```python
from build123d import *

# Parameters (mm, degrees)
F1_DEPTH = 2
F2_DEPTH = 4


with BuildPart() as f1:
    # F0 (on Top) → F1 (new body)
    with BuildSketch(Plane.XY):
        with BuildLine():
            ThreePointArc((32.5, 11.5), (31.035534, 15.035534), (27.5, 16.5))
            Line((27.5, 16.5), (-27.5, 16.5))
            ThreePointArc((-27.5, 16.5), (-31.035534, 15.035534), (-32.5, 11.5))
            Line((-32.5, 11.5), (-32.5, -11.5))
            ThreePointArc((-32.5, -11.5), (-31.035534, -15.035534), (-27.5, -16.5))
            Line((-27.5, -16.5), (27.5, -16.5))
            ThreePointArc((27.5, -16.5), (31.035534, -15.035534), (32.5, -11.5))
            Line((32.5, -11.5), (32.5, 11.5))
        make_face()
        with BuildLine():
            Line((-7.5, 14.5), (7.5, 14.5))
            ThreePointArc((7.5, 14.5), (11.035534, 13.035534), (12.5, 9.5))
            Line((12.5, 9.5), (12.5, -9.5))
            ThreePointArc((12.5, -9.5), (11.035534, -13.035534), (7.5, -14.5))
            Line((7.5, -14.5), (-7.5, -14.5))
            ThreePointArc((-7.5, -14.5), (-11.035534, -13.035534), (-12.5, -9.5))
            Line((-12.5, -9.5), (-12.5, 9.5))
            ThreePointArc((-12.5, 9.5), (-11.035534, 13.035534), (-7.5, 14.5))
        make_face(mode=Mode.SUBTRACT)
        with BuildLine():
            ThreePointArc((12.5, 9.5), (11.035534, 13.035534), (7.5, 14.5))
            Line((7.5, 14.5), (-7.5, 14.5))
            ThreePointArc((-7.5, 14.5), (-11.035534, 13.035534), (-12.5, 9.5))
            Line((-12.5, 9.5), (-12.5, -9.5))
            ThreePointArc((-12.5, -9.5), (-11.035534, -13.035534), (-7.5, -14.5))
            Line((-7.5, -14.5), (7.5, -14.5))
            ThreePointArc((7.5, -14.5), (11.035534, -13.035534), (12.5, -9.5))
            Line((12.5, -9.5), (12.5, 9.5))
        make_face()
        with BuildLine():
            Line((-4.5, 11), (4.5, 11))
            ThreePointArc((4.5, 11), (8.035534, 9.535534), (9.5, 6))
            Line((9.5, 6), (9.5, -6))
            ThreePointArc((9.5, -6), (8.035534, -9.535534), (4.5, -11))
            Line((4.5, -11), (-4.5, -11))
            ThreePointArc((-4.5, -11), (-8.035534, -9.535534), (-9.5, -6))
            Line((-9.5, -6), (-9.5, 6))
            ThreePointArc((-9.5, 6), (-8.035534, 9.535534), (-4.5, 11))
        make_face(mode=Mode.SUBTRACT)
    extrude(amount=F1_DEPTH)

    # F0 (on Top) → F2 (join)
    with BuildSketch(Plane.XY):
        with BuildLine():
            ThreePointArc((32.5, 11.5), (31.035534, 15.035534), (27.5, 16.5))
            Line((27.5, 16.5), (-27.5, 16.5))
            ThreePointArc((-27.5, 16.5), (-31.035534, 15.035534), (-32.5, 11.5))
            Line((-32.5, 11.5), (-32.5, -11.5))
            ThreePointArc((-32.5, -11.5), (-31.035534, -15.035534), (-27.5, -16.5))
            Line((-27.5, -16.5), (27.5, -16.5))
            ThreePointArc((27.5, -16.5), (31.035534, -15.035534), (32.5, -11.5))
            Line((32.5, -11.5), (32.5, 11.5))
        make_face()
        with BuildLine():
            Line((-7.5, 14.5), (7.5, 14.5))
            ThreePointArc((7.5, 14.5), (11.035534, 13.035534), (12.5, 9.5))
            Line((12.5, 9.5), (12.5, -9.5))
            ThreePointArc((12.5, -9.5), (11.035534, -13.035534), (7.5, -14.5))
            Line((7.5, -14.5), (-7.5, -14.5))
            ThreePointArc((-7.5, -14.5), (-11.035534, -13.035534), (-12.5, -9.5))
            Line((-12.5, -9.5), (-12.5, 9.5))
            ThreePointArc((-12.5, 9.5), (-11.035534, 13.035534), (-7.5, 14.5))
        make_face(mode=Mode.SUBTRACT)
    extrude(amount=F2_DEPTH)


solid = f1.part
```
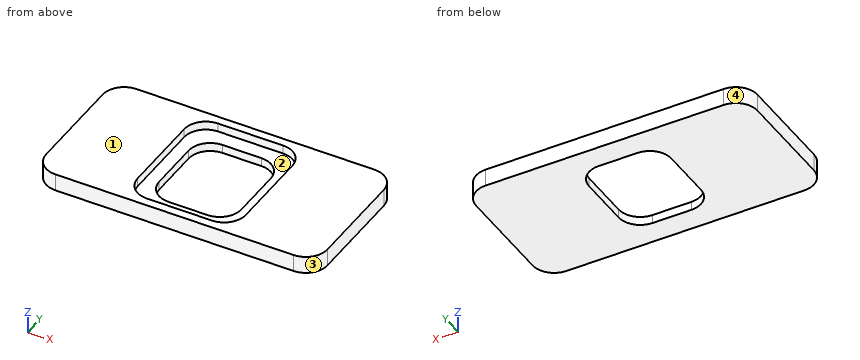
The model under review builds one solid part; all positions refer to its coordinate system, in mm. Face numbers are marked on the shaded views. Round coordinates to 2 decimals unless told otherwise and drop trailing zeros. Order: outer loops, then holes, each group sorted by start corner. A loop starts at its lowest first (then second) coordinate and runs counter-clockwise, first axis right, second up. Notation, with made-up numbers: (46.25, -17.5) -> (54.25, -17.5) arc R14 ccw to (54.25, -12.5) -> close; hole circle Ø10 at (-35, 27.25). An arc over 180 degrees is marked (long way). One line per item, written item: value. Start each with the question number.
Q1. Clearance check with flat-ended pins moving along their axes: pin 1 Ø10 at (x, y) = (6, -7.5) entering from +Z; pin 2 Ø1 at (x, y) = (6, -11) entering from -Z; pin 3 Ø8 at (x, y) = (-4, -6) entering from -Z. State where each tip first meets the part, or that it passes through.
Q2. Mouldability with a two-part tool opening along Y and no side actions: class the marked faces 1, 2, 3 and 4 as released by +Y, released by -Y, zero draft, split by the parting line, or undercut.
Q3. Take a section at A-A (z = 0.6). Write out the cut boundary in (x, y).
Q4. Take a section at B-B (y = 1.5). Write out the cut boundary in (x, z).
Q5. Take a section at D-D (x = -10.5). Write out the cut boundary in (y, z), and give its area (3 significant figures).
Q6. Wall thickness on line 1 (X direction, y = 0.5, z = 1.8); line 2 (X direction, y = 3.5, z = 3.2); line 3 (Y direction, x = 4, z = 2.85): over which ranges is each line inside the solid? List them lowest first.
Q7. Take a section at C-C (x = -1.5). Write out the cut boundary in (y, z).
Reported:
1. pin 1: stops at z = 2
1. pin 2: stops at z = 0
1. pin 3: passes through
2. face 1: zero draft
2. face 2: undercut
2. face 3: released by -Y
2. face 4: released by +Y
3. outline: (-32.5, -11.5) arc R5 ccw to (-27.5, -16.5) -> (27.5, -16.5) arc R5 ccw to (32.5, -11.5) -> (32.5, 11.5) arc R5 ccw to (27.5, 16.5) -> (-27.5, 16.5) arc R5 ccw to (-32.5, 11.5) -> close; hole (-9.5, -6) arc R5 ccw to (-4.5, -11) -> (4.5, -11) arc R5 ccw to (9.5, -6) -> (9.5, 6) arc R5 ccw to (4.5, 11) -> (-4.5, 11) arc R5 ccw to (-9.5, 6) -> close
4. outline: (-32.5, 0) -> (-9.5, 0) -> (-9.5, 2) -> (-12.5, 2) -> (-12.5, 4) -> (-32.5, 4) -> close; (9.5, 0) -> (32.5, 0) -> (32.5, 4) -> (12.5, 4) -> (12.5, 2) -> (9.5, 2) -> close
5. outline: (-16.5, 0) -> (16.5, 0) -> (16.5, 4) -> (13.5, 4) -> (13.5, 2) -> (-13.5, 2) -> (-13.5, 4) -> (-16.5, 4) -> close
5. area: 78.0 mm2
6. line 1: x = -32.5 to -9.5, 9.5 to 32.5
6. line 2: x = -32.5 to -12.5, 12.5 to 32.5
6. line 3: y = -16.5 to -14.5, 14.5 to 16.5
7. outline: (-16.5, 0) -> (-11, 0) -> (-11, 2) -> (-14.5, 2) -> (-14.5, 4) -> (-16.5, 4) -> close; (11, 0) -> (16.5, 0) -> (16.5, 4) -> (14.5, 4) -> (14.5, 2) -> (11, 2) -> close
